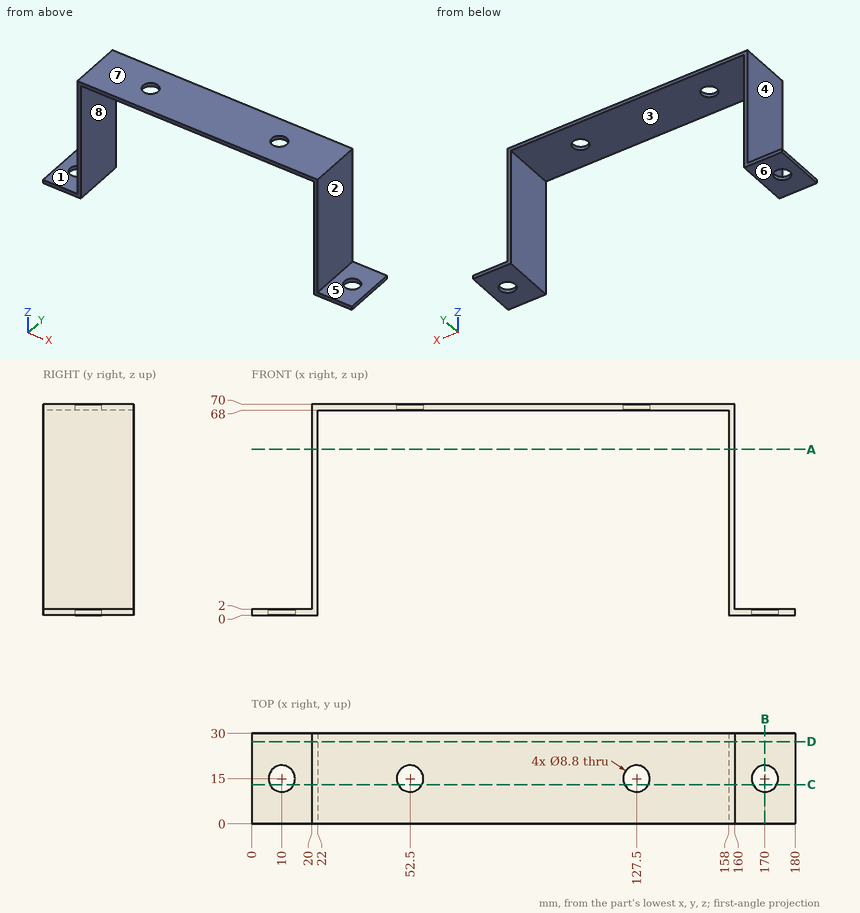
Input: dimensioned drawing with shaded views. Units: mm. Origin: part minimum x, y, z. A direction names the side the tool comes from. Give positions to 0.01 mm unless a question says otherwise; leave off trailing zeros. Write each loop counter-clockwise with the first axis right and the second up, starting at its lowest first coordinate (ties: lowest second). Pieces come first, ordered by that corner, then holes.
1. Material intervals for line 1 along X through (y, z) = (26.25, 16.5); line 2 along Z through (x, y) = (114, 11); line 3 along Z through (x, y) = (16, 23.75), sorted ascending.
2. Access query for the marked faces 4, 5, 6, 7 and 8. Directions: +Z, -Z, +X, -X, +Y, -Y. A direction counts if a zero-diameter tool reaches every point of the face in a straight line with its end or side. Return the directions, or none.
3. First-contact query: pin 1 (9 mm diameter, centred on y = 17, z = 43, fed in from -X); pin 2 (15 mm diameter, centred on y = 17.5, z = 50.5, fed in from +X); pin 3 (6 mm diameter, centred on x = 40, y = 11.5, fed in from -Z). Flat tips, straight axial feed; report the tip coordinate or a pass-through.
4. Section query C-C (y = 13). Return the cut outline in (x, z).
5. Section query B-B (x = 170). Return the cut outline in (y, z), then the cut area to 3 significant figures.
6. Section query A-A (z = 55). Return the cut outline in (x, y).
7. Pull-direction query (X, two-part tool) for the marked faces 1, 2 and 3; classes: +X half, -X half, draft (parallel to the pull), parting line (faces both ways), or undercut.
8. Section query D-D (y = 27.25). Return the cut outline in (x, z), then the cut area to 3 significant figures.
Output values:
1. line 1: x = 20 to 22, 158 to 160
1. line 2: z = 68 to 70
1. line 3: z = 0 to 2
2. face 4: +Z, -X, +Y, -Y
2. face 5: +Z, +X, +Y, -Y
2. face 6: -Z, +X, -X, +Y, -Y
2. face 7: +Z, +X, -X, +Y, -Y
2. face 8: -Z, +Y, -Y
3. pin 1: stops at x = 20
3. pin 2: stops at x = 160
3. pin 3: stops at z = 68
4. outline: (0, 0) - (6.08, 0) - (6.08, 2) - (0, 2) - close; (13.92, 0) - (22, 0) - (22, 68) - (48.58, 68) - (48.58, 70) - (20, 70) - (20, 2) - (13.92, 2) - close; (56.42, 68) - (123.58, 68) - (123.58, 70) - (56.42, 70) - close; (131.42, 68) - (158, 68) - (158, 0) - (166.08, 0) - (166.08, 2) - (160, 2) - (160, 70) - (131.42, 70) - close; (173.92, 0) - (180, 0) - (180, 2) - (173.92, 2) - close
5. outline: (0, 0) - (10.6, 0) - (10.6, 2) - (0, 2) - close; (19.4, 0) - (30, 0) - (30, 2) - (19.4, 2) - close
5. area: 42.4 mm2
6. outline: (20, 0) - (22, 0) - (22, 30) - (20, 30) - close; (158, 0) - (160, 0) - (160, 30) - (158, 30) - close
7. face 1: draft
7. face 2: +X half
7. face 3: undercut
8. outline: (0, 0) - (22, 0) - (22, 68) - (158, 68) - (158, 0) - (180, 0) - (180, 2) - (160, 2) - (160, 70) - (20, 70) - (20, 2) - (0, 2) - close
8. area: 632 mm2
